Could you check a few things on this drawing? It's one solid part, dimensions in mm from its lowest x, y, z. A direction names the side the tool comes from. Give positions to 0.01 mm unless a question says otherwise; leave off trailing zeros. Write each loop counter-clockwise with the first axis right and the second up, starting at its lowest first coordinate (ties: lowest second). Pieces come first, ordered by that corner, then holes. Notation, with made-up numbers: M 81.25,-5 L 88.25,-5 A24 cw 88.25,27 Z; hole C 31,-7.5 d5. An arc over 180 degrees is marked long. Use CSV: the item, a comma, the result in double quotes. Start each with the question number.
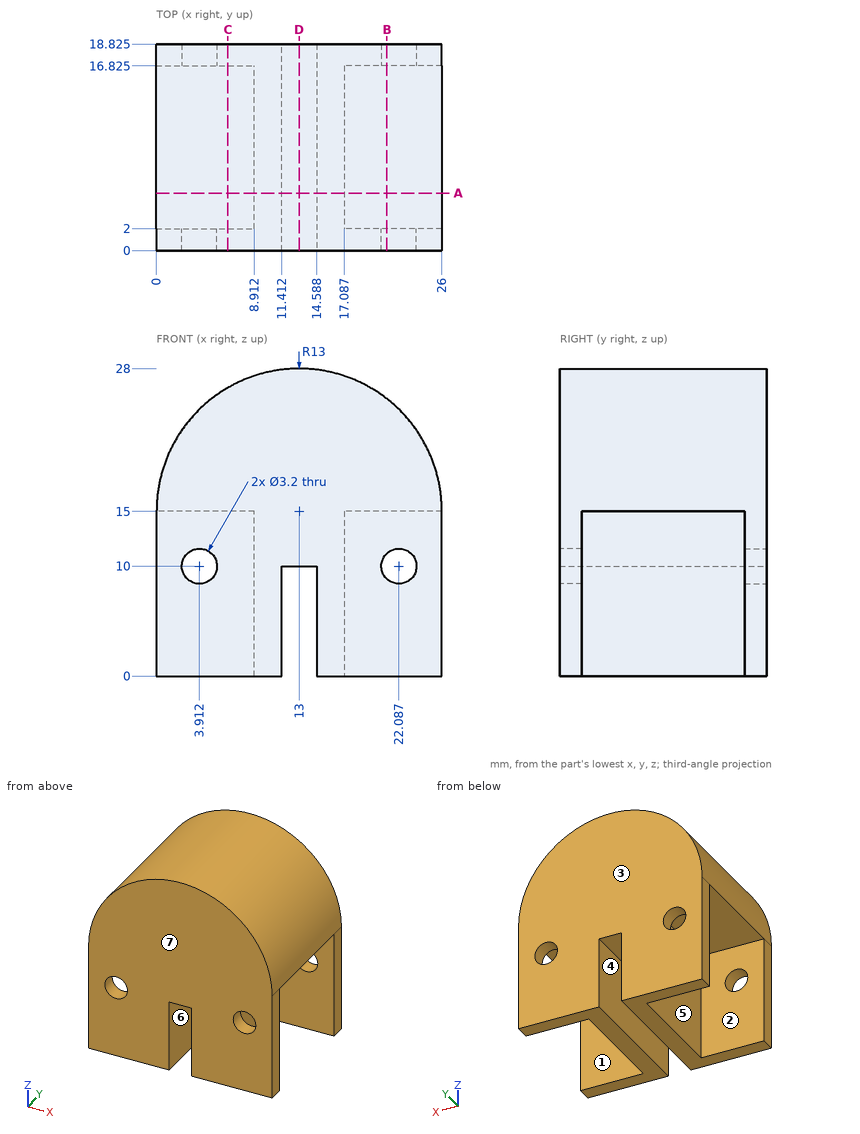
(1) Thinking about a two-plate mould opening in Y: for the marked faces 5, 6 and 7, which applies, released by +Y, released by -Y, zero draft, split by the parting line, or undercut?
(2) Which directions (+Z, -Z, +X, -X, +Y, -Y) give clear straight access to the entire face, cutting with the end or side of a thin tool? Please do the marked faces 1, 2, 3 and 4.
(3) I want a section at B-B (x = 21). Write out the boundary of the cut face in (y, z) (1 decimal).
(4) I want a section at A-A (y = 5.25). Write out the boundary of the cut face in (x, z).
(5) I want a section at C-C (x = 6.5). Write out the boundary of the cut face in (y, z) (1 decimal).
(6) I want a section at D-D (x = 13). Write out the boundary of the cut face in (y, z) (1 decimal).
(7) Please list where these lines run through material, in increasing order: L1, parallel to Y at x = 18.25, z = 13.25 (1 decimal); L2, parallel to X at y = 16.75, z = 3; L3, parallel to X at y = 16.5, z = 13.5. Write a range as [from, to].
(8) Will these pins go through, and if not, where does the flat tip stop? pin 1 Ø3 at (y, z) = (11, 7) entering from -X; pin 2 Ø1 at (x, y) = (13, 10.5) entering from -Z; pin 3 Ø1 at (x, y) = (19.5, 8.5) entering from +Z; pin 4 Ø3 at (x, z) = (22.09, 10) entering from -Y.
Geometry results:
1,face 5,"undercut"
1,face 6,"zero draft"
1,face 7,"released by -Y"
2,face 1,"-Z, +X"
2,face 2,"-Z, -X"
2,face 3,"+Z, -Z, +X, -X, +Y"
2,face 4,"-Z, +Y, -Y"
3,outline,"M 0,0 L 2,0 L 2,8.8 L 0,8.8 Z; M 0,11.2 L 2,11.2 L 2,15 L 16.8,15 L 16.8,11.2 L 18.8,11.2 L 18.8,25.2 L 0,25.2 Z; M 16.8,0 L 18.8,0 L 18.8,8.8 L 16.8,8.8 Z"
4,outline,"M 0,15 L 8.91,15 L 8.91,0 L 11.41,0 L 11.41,10 L 14.59,10 L 14.59,0 L 17.09,0 L 17.09,15 L 26,15 A13 ccw Z"
5,outline,"M 0,0 L 2,0 L 2,15 L 16.8,15 L 16.8,0 L 18.8,0 L 18.8,26.3 L 0,26.3 Z"
6,outline,"M 0,10 L 18.8,10 L 18.8,28 L 0,28 Z"
7,L1,"y = [0, 2], [16.8, 18.8]"
7,L2,"x = [8.91, 11.41], [14.59, 17.09]"
7,L3,"x = [8.91, 17.09]"
8,pin 1,"stops at x = 8.91"
8,pin 2,"stops at z = 10"
8,pin 3,"stops at z = 26.53"
8,pin 4,"passes through"
